Here's the drawing with two shaded views (mm, measured from the low corner). I have some questions. Give positions to 0.01 mm unless a question says otherwise; leave off trailing zeros. Loops run counter-clockwise (first coordinate to the right, second up) from the corner with the lowest first, then second, coordinate; pieces in that order, holes last.
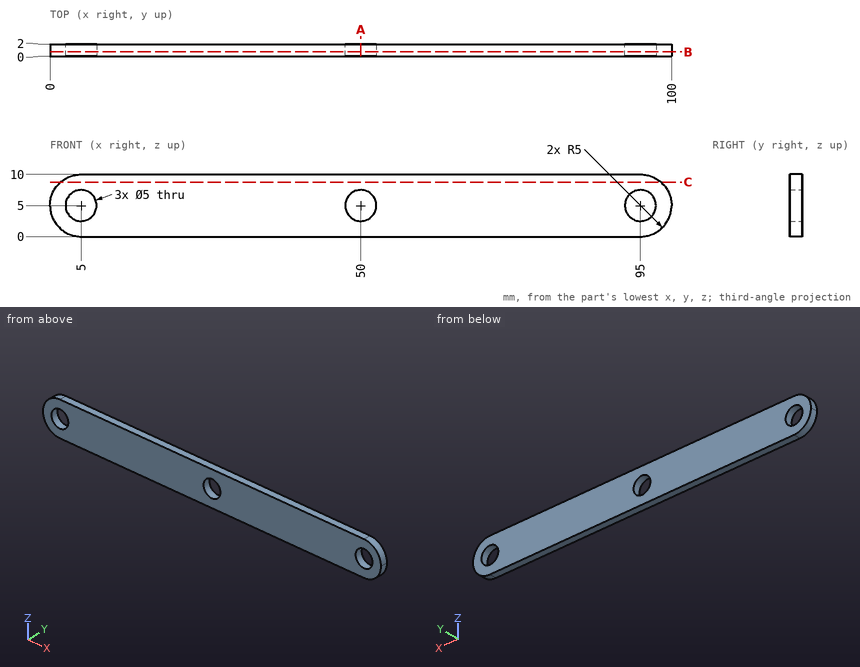
(1) Suppose I cut it at A-A on x = 50. List the corners of the cut face in (y, z) for me.
Returned:
outline: (0, 0) - (2, 0) - (2, 2.5) - (0, 2.5) - close; (0, 7.5) - (2, 7.5) - (2, 10) - (0, 10) - close
(2) Suppose I cut it at C-C on z = 8.75. List the corners of the cut face in (x, y) for me, plus the area to 3 significant figures.
Returned:
outline: (1.69, 0) - (98.31, 0) - (98.31, 2) - (1.69, 2) - close
area: 193 mm2
(3) Suppose I cut it at B-B on y = 0.75. Give the number of separate pieces and of enclosed holes in the cut face, plus the area to 3 significant figures.
Returned:
separate pieces: 1
enclosed holes: 3
area: 920 mm2
(4) Please list where these lines run through material, in increasing order: probe 1 along Z at (x, y) = (95, 1.3); probe 2 along X at (y, z) = (1.3, 7.25); probe 3 along X at (y, z) = (0.4, 6.25).
Returned:
probe 1: z = 0 to 2.5, 7.5 to 10
probe 2: x = 0.53 to 3.91, 6.09 to 48.91, 51.09 to 93.91, 96.09 to 99.47
probe 3: x = 0.16 to 2.83, 7.17 to 47.83, 52.17 to 92.83, 97.17 to 99.84
